from build123d import *

# Parameters (mm, degrees)
BOSS_EXTRUDE1_DEPTH   = 30
SKETCH4_R             = 2
CUT_EXTRUDE1_DEPTH    = 10
LPATTERN9_COUNT       = 4
LPATTERN9_PITCH       = 19
SKETCH5_W             = 9.377010815
SKETCH5_H             = 30
BOSS_EXTRUDE2_DEPTH   = 2
SKETCH5_W_2           = 8.706514496
BOSS_EXTRUDE2_2_DEPTH = 2
SKETCH6_R             = 1.75
CUT_EXTRUDE2_DEPTH    = 81.473598155
BOSS_EXTRUDE4_DEPTH   = 3
SKETCH10_W            = 1.262251727
SKETCH10_H            = 1.617260026
CUT_EXTRUDE3_DEPTH    = 55
SKETCH11_R            = 1.75
BOSS_EXTRUDE5_DEPTH   = 3


# Read off the part's stored shape, not the designer's step: Boundary-Cut1
with BuildPart() as part:
    # Sketch1 → Boss-Extrude1 (new body)
    with BuildSketch(Plane(origin=(0, 0, 0), x_dir=(1, 0, 0), z_dir=(0, 1, 0))):
        with BuildLine():
            Line((-10, 0), (10, 0))
            ThreePointArc((10, 0), (0, 10), (-10, 0))
        make_face()
    boss_extrude1 = extrude(amount=BOSS_EXTRUDE1_DEPTH)

    # Boundary-Cut1 outline → Boundary-Cut1 (revolve, cut)
    with BuildSketch(Plane.XY):
        Polygon((0, 30.000006646), (0, 5), (5, 5), (6.500000399, 30.000006646), align=None)
    boundary_cut1 = revolve(axis=Axis((0, 0, 0), (0, 1, 0)), mode=Mode.SUBTRACT)

    # Sketch4 → Cut-Extrude1 (cut)
    with BuildSketch(Plane(origin=(0, 5, 0), x_dir=(1, 0, 0), z_dir=(0, 1, 0))):
        Circle(SKETCH4_R)
    cut_extrude1 = extrude(amount=-CUT_EXTRUDE1_DEPTH, mode=Mode.SUBTRACT)

    # LPattern9: Boss-Extrude1, Boundary-Cut1, Cut-Extrude1 ×4
    with Locations(*[(i * LPATTERN9_PITCH, 0, 0) for i in range(1, LPATTERN9_COUNT)]):
        add(boss_extrude1)
        add(boundary_cut1, mode=Mode.SUBTRACT)
        add(cut_extrude1, mode=Mode.SUBTRACT)



with BuildPart() as body_2:
    # Sketch5 → Boss-Extrude2 (new body)
    with BuildSketch(Plane.XY):
        with Locations((-12.311494593, 15)):
            Rectangle(SKETCH5_W, SKETCH5_H)
    extrude(amount=-BOSS_EXTRUDE2_DEPTH)


with BuildPart() as body_3:
    # Sketch5 → Boss-Extrude2 2 (new body)
    with BuildSketch(Plane.XY):
        with Locations((69.646742752, 15)):
            Rectangle(SKETCH5_W_2, SKETCH5_H)
    extrude(amount=-BOSS_EXTRUDE2_2_DEPTH)


with BuildPart() as cut_extrude2_tool:
    # Sketch6 → Cut-Extrude2 (new, through all)
    with BuildSketch(Plane.XY):
        with Locations((-13.5, 23)):
            Circle(SKETCH6_R)
        with Locations((-13.5, 7)):
            Circle(SKETCH6_R)
        with Locations((70.5, 23)):
            Circle(SKETCH6_R)
        with Locations((70.5, 7)):
            Circle(SKETCH6_R)
    extrude(amount=-CUT_EXTRUDE2_DEPTH)


with BuildPart() as body_2_1:
    add(body_2.part)

    # Cut-Extrude2: cut by cut_extrude2_tool
    add(cut_extrude2_tool.part, mode=Mode.SUBTRACT)


with BuildPart() as body_3_1:
    add(body_3.part)

    # Cut-Extrude2: cut by cut_extrude2_tool
    add(cut_extrude2_tool.part, mode=Mode.SUBTRACT)


with BuildPart() as part_1:
    add(part.part)

    add(body_2_1.part)  # Boss-Extrude4 merges body 2

    add(body_3_1.part)  # Boss-Extrude4 merges body 3
    # Sketch9 → Boss-Extrude4 (add)
    with BuildSketch(Plane.XZ):
        with BuildLine():
            Line((5, 0), (14, 0))
            ThreePointArc((14, 0), (19, -5), (24, 0))
            Line((24, 0), (33, 0))
            ThreePointArc((33, 0), (38, -5), (43, 0))
            Line((43, 0), (52, 0))
            ThreePointArc((52, 0), (57, -5), (62, 0))
            Line((62, 0), (67, 0))
            Line((67, 0), (74, 0))
            Line((74, 0), (74, -2))
            Line((74, -2), (66.94427191, -2))
            ThreePointArc((66.94427191, -2), (64, -7.708203932), (58, -10))
            Line((58, -10), (-1, -10))
            ThreePointArc((-1, -10), (-7, -7.708203932), (-9.94427191, -2))
            Line((-9.94427191, -2), (-17, -2))
            Line((-17, -2), (-17, 0))
            Line((-17, 0), (-10, 0))
            Line((-10, 0), (-5, 0))
            ThreePointArc((-5, 0), (0, -5), (5, 0))
        make_face()
    extrude(amount=BOSS_EXTRUDE4_DEPTH)

    # Sketch10 → Cut-Extrude3 (cut)
    with BuildSketch(Plane(origin=(0, 0, 0), x_dir=(0, 0, -1), z_dir=(1, 0, 0))):
        with Locations((-0.197226833, 7.234540745)):
            Rectangle(SKETCH10_W, SKETCH10_H)
    extrude(amount=CUT_EXTRUDE3_DEPTH, mode=Mode.SUBTRACT)

    # Sketch11 → Boss-Extrude5 (add)
    with BuildSketch(Plane.XY):
        with BuildLine():
            Line((25.500111158, 30), (31.499888841, 30))
            Line((31.499888841, 30), (31.499888841, 35))
            ThreePointArc((31.499888841, 35), (31.206995622, 35.707106781), (30.499888841, 36))
            Line((30.499888841, 36), (26.500111158, 36))
            ThreePointArc((26.500111158, 36), (25.793004377, 35.707106781), (25.500111158, 35))
            Line((25.500111158, 35), (25.500111158, 30))
        make_face()
        with Locations((28.5, 33)):
            Circle(SKETCH11_R, mode=Mode.SUBTRACT)
    extrude(amount=-BOSS_EXTRUDE5_DEPTH)


solid = part_1.part
Could you check a few things on this model? Use its own coordinates, in mm. A direction names the side the tool comes from. Give positions to 0.01 mm unless a question says otherwise; leave off trailing zeros. Order: outer loops, then holes, each group sorted by start corner. A loop starts at its lowest first (then second) coordinate and runs counter-clockwise, first axis right, second up.
1. For pin 1 (4 mm diameter, centred on x = 16.5, z = -1.5, fed in from -Y); pin 2 (3 mm diameter, centred on x = 70.5, y = 7, fed in from +Z); pin 3 (4 mm diameter, centred on x = 31.5, y = 13.5, fed in from -Z); pin 4 (2.5 mm diameter, centred on x = 57.5, z = -2.5, fed in from +Y), each with a flat end and sliding along its axis, tell me the tip position at first contact or that it passes through.
Answers below:
pin 1: stops at y = 0
pin 2: passes through
pin 3: stops at z = -8.93
pin 4: stops at y = 5
2. Which directions (+Z, -Z, +X, -X, +Y, -Y) give clear straight access to the entire face, cutting with the end or side of a thin tool? Please do faces 5 (the flat face through (57, 5, -3)), 6 (the cylindrical face through (0, -1, -5)), 7 (the flat face through (27.1, 31.7, -3)).
Answers below:
face 5: +Z, +Y
face 6: +Z, -Y
face 7: -Z, +X, -X, +Y
3. I need wall thicknesses on L1, parallel to Y at x = 70.5, z = -0.55; L2, parallel to X at y = 21, z = -1.5; L3, parallel to X at y = 1, z = -6.5. Which ranges of each line are inside material? Lowest first, please.
Answers below:
L1: y = -3 to 5.25, 8.75 to 21.25, 24.75 to 30
L2: x = -17 to -5.77, 5.77 to 13.23, 24.77 to 32.23, 43.77 to 51.23, 62.77 to 74
L3: x = -7.6 to 7.6, 11.4 to 26.6, 30.4 to 45.6, 49.4 to 64.6
4. Suppose I cut it at D-D (y = 23). Write out the boundary of the cut face in (x, z).
Answers below:
outline: (-17, -2) - (-15.25, -2) - (-15.25, 0) - (-17, 0) - close; (-11.75, -2) - (-9.8, -2) arc R10 ccw to (9.5, -3.12) arc R10 ccw to (28.5, -3.12) arc R10 ccw to (47.5, -3.12) arc R10 ccw to (66.8, -2) - (68.75, -2) - (68.75, 0) - (63.08, 0) arc R6.08 cw to (50.92, 0) - (44.08, 0) arc R6.08 cw to (31.92, 0) - (25.08, 0) arc R6.08 cw to (12.92, 0) - (6.08, 0) arc R6.08 cw to (-6.08, 0) - (-11.75, 0) - close; (72.25, -2) - (74, -2) - (74, 0) - (72.25, 0) - close
5. Thinking about a two-plate mould opening in X: for faces 1 (the flat face through (64.2, 0, -7.2)), 2 (the conical face through (19.13, 17.67, -5.76)), 3 (the cylindrical face through (38, -1, -5)), 4 (the cylindrical face through (-6.93, -1.48, -7.77)), which applies, +X half, -X half, draft (parallel to the pull), parting line (faces both ways), or undercut?
Answers below:
face 1: draft
face 2: undercut
face 3: undercut
face 4: -X half
6. Suppose I cut it at A-A (x = -13.5). Write out the boundary of the cut face in (y, z), plus the area to 3 significant figures.
Answers below:
outline: (-3, -2) - (5.25, -2) - (5.25, 0) - (-3, 0) - close; (8.75, -2) - (21.25, -2) - (21.25, 0) - (8.75, 0) - close; (24.75, -2) - (30, -2) - (30, 0) - (24.75, 0) - close
area: 52.0 mm2
7. Suppose I cut it at B-B (y = 18.5). Write out the boundary of the cut face in (x, z), plus the area to 3 significant figures.
Answers below:
outline: (-17, -2) - (-9.8, -2) arc R10 ccw to (9.5, -3.12) arc R10 ccw to (28.5, -3.12) arc R10 ccw to (47.5, -3.12) arc R10 ccw to (66.8, -2) - (74, -2) - (74, 0) - (62.81, 0) arc R5.81 cw to (51.19, 0) - (43.81, 0) arc R5.81 cw to (32.19, 0) - (24.81, 0) arc R5.81 cw to (13.19, 0) - (5.81, 0) arc R5.81 cw to (-5.81, 0) - (-17, 0) - close
area: 438 mm2
8. Suppose I cut it at C-C (y = 33). Write out the boundary of the cut face in (x, z), plus the area to 3 significant figures.
Answers below:
outline: (25.5, -3) - (26.75, -3) - (26.75, 0) - (25.5, 0) - close; (30.25, -3) - (31.5, -3) - (31.5, 0) - (30.25, 0) - close
area: 7.50 mm2
